Can you work these out from the model? Positions are in its coordinate system, mm. Face numbers are marked on the shaded views. A direction names the side the tool comes from. Round coordinates to 2 decimals unless told otherwise and drop trailing zeros. Loops run counter-clockwise (first coordinate to the right, second up) from the corner with the lowest first, then second, coordinate; pieces in that order, holes last. Notation, with made-up numbers: (39.25, 75.5) -> (61.25, 75.5) arc R20 cw to (61.25, 114.5) -> close; hole circle Ø8 at (-32.5, 29). An arc over 180 degrees is marked (long way). Answer as a JSON object with one key per item and string values.
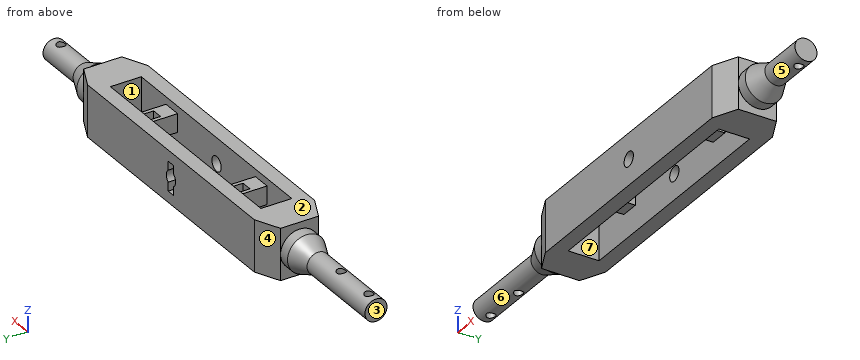
```python
from build123d import *

# Parameters (mm, degrees)
SKETCH1_W                   = 32.5
SKETCH1_H                   = 4.2
BASEFORM_DEPTH              = 7
SKETCH2_R                   = 1
HUMERUSAXLEHOLE1_DEPTH      = 2
HUMERUSAXLELOCK_DEPTH       = 1
SKETCH6_R                   = 1.5
AXLEEXTENSION_DEPTH         = 6
SKETCH7_R                   = 0.6
SCREWHOLES_DEPTH            = 54.273445543
SCREWHOLES_DEPTH_BACK       = 54.273445543
SKETCH8_W                   = 2.5
SKETCH8_H                   = 2.5
HUMERUSTUBEHOLDERBASE_DEPTH = 4.2
SKETCH13_W                  = 1.5
SKETCH13_H                  = 1.5
TUBECLIPENTRANCE_DEPTH      = 2
SKETCH14_W                  = 1.5
SKETCH14_H                  = 1.5
CABLECLIPLOCKSLOT_DEPTH     = 0.7
SKETCH15_W                  = 1.5
SKETCH15_H                  = 0.2
TUBECLIPLOCKCLEARANCE_DEPTH = 2
SKETCH12_R                  = 1
HUMERUSAXLEHOLE2_DEPTH      = 54.818584249


with BuildPart() as part:
    # Sketch1 → BaseForm (new body)
    with BuildSketch(Plane.XY):
        Polygon((0, -2.584500111), (0, 2.584500111), (3.25, 4.1), (39.25, 4.1), (42.5, 2.584500111), (42.5, -2.584500111), (39.25, -4.1), (3.25, -4.1), align=None)
        with Locations((21.25, 0)):
            Rectangle(SKETCH1_W, SKETCH1_H, mode=Mode.SUBTRACT)
    extrude(amount=BASEFORM_DEPTH)

    # Sketch2 → HumerusAxleHole1 (cut)
    with BuildSketch(Plane(origin=(0, 4.1, 0), x_dir=(1, 0, 0), z_dir=(0, 1, 0))):
        with Locations(Location((21.25, -3.5, 0), (0, 0, 270))):
            Circle(SKETCH2_R)
    extrude(amount=-HUMERUSAXLEHOLE1_DEPTH, mode=Mode.SUBTRACT)

    # Sketch2_4 → HumerusAxleLock (cut)
    with BuildSketch(Plane(origin=(0, 4.1, 0), x_dir=(1, 0, 0), z_dir=(0, 1, 0))):
        with BuildLine():
            ThreePointArc((20.65, -2.7), (21.25, -2.5), (21.85, -2.7))
            Line((21.85, -2.7), (21.85, -1.5))
            Line((21.85, -1.5), (20.65, -1.5))
            Line((20.65, -1.5), (20.65, -2.7))
        make_face()
        with BuildLine():
            Line((21.85, -5.5), (21.85, -4.3))
            ThreePointArc((21.85, -4.3), (21.25, -4.5), (20.65, -4.3))
            Line((20.65, -4.3), (20.65, -5.5))
            Line((20.65, -5.5), (21.85, -5.5))
        make_face()
    extrude(amount=-HUMERUSAXLELOCK_DEPTH, mode=Mode.SUBTRACT)

    # Sketch5 → Axle (revolve)
    with BuildSketch(Plane.XY.offset(3.5), mode=Mode.PRIVATE) as axle_sk:
        Polygon((53, 0), (53, 1.5), (46.5, 1.5), (44, 2.584500111), (42.5, 2.584500111), (42.5, 0), align=None)
    axle = revolve(axle_sk.sketch.rotate(Axis((42.5, 0, 3.5), (1, 0, 0)), 90), axis=Axis((42.5, 0, 3.5), (1, 0, 0)))

    # Axle2: Axle across plane
    add(axle.mirror(Plane.ZY.offset(-21.25)))

    # Sketch6 → AxleExtension (add)
    with BuildSketch(Plane.ZY.offset(10.5)):
        with Locations((3.5, 0)):
            Circle(SKETCH6_R)
    extrude(amount=AXLEEXTENSION_DEPTH)

    # Sketch7 → ScrewHoles (cut, two sides)
    with BuildSketch(Plane.XY.offset(3.5)) as screwholes_sk:
        with Locations((-9, 0)):
            Circle(SKETCH7_R)
        with Locations((-15, 0)):
            Circle(SKETCH7_R)
        with Locations((51.5, 0)):
            Circle(SKETCH7_R)
    extrude(amount=SCREWHOLES_DEPTH, mode=Mode.SUBTRACT)
    extrude(screwholes_sk.sketch, amount=-SCREWHOLES_DEPTH_BACK, mode=Mode.SUBTRACT)

    # Sketch8 → HumerusTubeHolderBase (add)
    with BuildSketch(Plane(origin=(0, 2.1, 0), x_dir=(1, 0, 0), z_dir=(0, 1, 0))):
        with Locations((11.6, -4.75)):
            Rectangle(SKETCH8_W, SKETCH8_H)
    humerustubeholderbase = extrude(amount=-HUMERUSTUBEHOLDERBASE_DEPTH)

    # Sketch13 → TubeClipEntrance (cut)
    with BuildSketch(Plane.XY.offset(6)):
        with Locations((11.6, 0.65)):
            Rectangle(SKETCH13_W, SKETCH13_H)
    tubeclipentrance = extrude(amount=-TUBECLIPENTRANCE_DEPTH, mode=Mode.SUBTRACT)

    # Sketch14 → CableClipLockSlot (cut)
    with BuildSketch(Plane.XZ.offset(-1.4)):
        with Locations((11.6, 4.75)):
            Rectangle(SKETCH14_W, SKETCH14_H)
    cablecliplockslot = extrude(amount=-CABLECLIPLOCKSLOT_DEPTH, mode=Mode.SUBTRACT)

    # Sketch15 → TubeClipLockClearance (cut)
    with BuildSketch(Plane.XY.offset(6)):
        with Locations((11.6, 1.5)):
            Rectangle(SKETCH15_W, SKETCH15_H)
    tubecliplockclearance = extrude(amount=-TUBECLIPLOCKCLEARANCE_DEPTH, mode=Mode.SUBTRACT)

    # Sketch12 → HumerusAxleHole2 (cut, through all)
    with BuildSketch(Plane(origin=(0, -2.1, 0), x_dir=(1, 0, 0), z_dir=(0, 1, 0))):
        with Locations(Location((21.25, -3.5, 0), (0, 0, 306.869897646))):
            Circle(SKETCH12_R)
    extrude(amount=-HUMERUSAXLEHOLE2_DEPTH, mode=Mode.SUBTRACT)

    # TubeClipSlot2: HumerusTubeHolderBase, TubeClipEntrance, CableClipLockSlot, TubeClipLockClearance across plane
    add(humerustubeholderbase.mirror(Plane(origin=(21.25, 0, 0), x_dir=(0, 0, 1), z_dir=(1, 0, 0))))
    add(tubeclipentrance.mirror(Plane(origin=(21.25, 0, 0), x_dir=(0, 0, 1), z_dir=(1, 0, 0))), mode=Mode.SUBTRACT)
    add(cablecliplockslot.mirror(Plane(origin=(21.25, 0, 0), x_dir=(0, 0, 1), z_dir=(1, 0, 0))), mode=Mode.SUBTRACT)
    add(tubecliplockclearance.mirror(Plane(origin=(21.25, 0, 0), x_dir=(0, 0, 1), z_dir=(1, 0, 0))), mode=Mode.SUBTRACT)


solid = part.part
```
Q1. On a 3-axis mill with a long thin cutter (end or side, diameter ignored), from which of +Z, -Z, +X, -X, +Y, -Y can I reach the whole of each face in a straight line? I mean the marked faces 4, 5, 6 and 7. Say none if no direction works.
Determined:
{"face 4": "+Z, -Z, -X, +Y", "face 5": "+X", "face 6": "-X", "face 7": "+Z, -Z"}
Q2. We'd pull the mould along X, two halves only. Please class the marked faces 1, 2 and 3: pulls with the +X half, pulls with the -X half, needs draft (parallel to the pull), parting line crosses it, or undercut.
Determined:
{"face 1": "undercut", "face 2": "needs draft", "face 3": "pulls with the -X half"}
Q3. I want a section at B-B, the plane x = -15. Write out the boundary of the cut face in (y, z).
Determined:
{"outline": "(-0.6, 2.13) -> (-0.6, 4.87) arc R1.5 ccw to start; (0.6, 2.13) arc R1.5 ccw to (0.6, 4.87) -> close"}
Q4. I'm going to push flat-ended pins straight in: pin 1 (4 mm diameter, centred on x = -8, z = 3.5, fed in from -Y); pin 2 (1 mm diameter, centred on y = 0.5, z = 1.5, fed in from +X); pin 3 (0.5 mm diameter, centred on x = 30.5, y = 1.5, fed in from +Z). Where does each tip first touch, or does it pass through?
Determined:
{"pin 1": "y = -1.5", "pin 2": "x = 46.36", "pin 3": "z = 6"}
Q5. I want a section at A-A, the plane x = 21.25. Write out the boundary of the cut face in (y, z), then the cut area to 3 significant figures.
Determined:
{"outline": "(-4.1, 0) -> (-2.1, 0) -> (-2.1, 2.5) -> (-4.1, 2.5) -> close; (-4.1, 4.5) -> (-2.1, 4.5) -> (-2.1, 7) -> (-4.1, 7) -> close; (2.1, 0) -> (4.1, 0) -> (4.1, 1.5) -> (3.1, 1.5) -> (3.1, 2.5) -> (2.1, 2.5) -> close; (2.1, 4.5) -> (3.1, 4.5) -> (3.1, 5.5) -> (4.1, 5.5) -> (4.1, 7) -> (2.1, 7) -> close", "area": "18.0 mm²"}
Q6. If I drill on L1, parallel to X at y = 0, z = 3.1; L2, parallel to X at y = 2, z = 0.75; L3, parallel to Y at x = 20, z = 6, over which ranges is the centre line in solid material (lowest first)? Write a range as [from, to].
Determined:
{"L1": "[-16.5, -15.6], [-14.4, -9.6], [-8.4, 5], [37.5, 50.9], [52.1, 53]", "L2": "[0, 5], [37.5, 42.5]", "L3": "[-4.1, -2.1], [2.1, 4.1]"}
